Source: CAD feature listing. Evaluate the final solid. Frame: model axes, mm. Give positions to 0.01 mm unless a question says otherwise; leave off trailing zeros. Order: outer loops, then holes, each group sorted by start corner. A loop starts at its lowest first (then second) coordinate and runs counter-clockwise, first axis right, second up. Notation, with made-up numbers: (51.5, 56) - (62.5, 56) arc R25 cw to (62.5, 94) - close; hole circle Ø10 at (41, 42.5). An arc over 180 degrees is marked (long way). Write each question's results on one line, items separated by ' | '. Start each with the question number.
Item 1: Section C-C on y = 1139. Output: boundary loops of the cut face in (x, z), and give its area (3 significant figures).
Item 2: Contact query for flat-ended pins moving along their axis: pin 1 Ø2 at (x, y) = (5.5, 1030.5) entering from +Z; pin 2 Ø1.2 at (x, y) = (0.5, 1124) entering from -Z; pin 3 Ø1.2 at (y, z) = (1205.5, -1) entering from -X; pin 4 Ø1.6 at (x, z) = (1, -10) entering from +Y. Output: stop coordinate, or through.
Item 3: Section B-B on z = -8.75. Output: boundary loops of the cut face in (x, y), and give its area (4 significant figures).
Item 4: Section A-A on x = 4.5. Output: boundary loops of the cut face in (y, z).
Item 5: Line query: line 1 along X through (y, z) = (980, -14.5); line 2 along Z through (x, y) = (12, 1135.5); line 3 along Y through (x, z) = (4.5, -1). Output: solid intervals per line, ascending.
```python
from build123d import *

# Parameters (mm, degrees)
SKETCH1_W                   = 17
SKETCH1_H                   = 17
BOSS_EXTRUDE1_DEPTH         = 1220
CUT_EXTRUDE1_START          = -20
SKETCH2_W                   = 20
SKETCH2_H                   = 20
CUT_EXTRUDE1_DEPTH          = 10
CUT_EXTRUDE2_DEPTH          = 15
SKETCH4_W                   = 3
SKETCH4_H                   = 10
CUT_EXTRUDE3_DEPTH          = 10
SKETCH_PATTERN1_START       = -20
SKETCH_PATTERN1_DEPTH       = 15
SKETCH_PATTERN1_2_OUTLINE_W = 1.5
SKETCH_PATTERN1_2_OUTLINE_H = 10
SKETCH_PATTERN1_2_DEPTH     = 3
SKETCH6_W                   = 20
SKETCH6_H                   = 785
CUT_EXTRUDE4_DEPTH          = 1221.327824808


# Read off the part's stored shape, not the designer's step: Sketch-Pattern1
with BuildPart() as part:
    # Sketch1 → Boss-Extrude1 (new body)
    with BuildSketch(Plane(origin=(0, 0, 0), x_dir=(1, 0, 0), z_dir=(0, 1, 0))):
        with BuildLine():
            Line((0.5, 0), (19.5, 0))
            ThreePointArc((19.5, 0), (19.853553391, 0.146446609), (20, 0.5))
            Line((20, 0.5), (20, 19.5))
            ThreePointArc((20, 19.5), (19.853553391, 19.853553391), (19.5, 20))
            Line((19.5, 20), (0.5, 20))
            ThreePointArc((0.5, 20), (0.146446609, 19.853553391), (0, 19.5))
            Line((0, 19.5), (0, 0.5))
            ThreePointArc((0, 0.5), (0.146446609, 0.146446609), (0.5, 0))
        make_face()
        with Locations((10, 10)):
            Rectangle(SKETCH1_W, SKETCH1_H, mode=Mode.SUBTRACT)
    extrude(amount=BOSS_EXTRUDE1_DEPTH)

    # Sketch2 → Cut-Extrude1 (cut)
    with BuildSketch(Plane(origin=(20, 0, 0), x_dir=(0, 0, -1), z_dir=(1, 0, 0)).offset(CUT_EXTRUDE1_START)):
        with Locations((10, 1210)):
            Rectangle(SKETCH2_W, SKETCH2_H)
        with Locations((10, 10)):
            Rectangle(SKETCH2_W, SKETCH2_H)
    extrude(amount=CUT_EXTRUDE1_DEPTH, mode=Mode.SUBTRACT)

    # Sketch3 → Cut-Extrude2 (cut)
    with BuildSketch(Plane(origin=(0, 0, -20), x_dir=(-1, 0, 0), z_dir=(0, 0, -1))):
        Polygon((-15, 1115), (0, 1115), (0, 1120), (-9, 1120), (-9, 1130), (0, 1130), (0, 1135), (-15, 1135), align=None)
    extrude(amount=-CUT_EXTRUDE2_DEPTH, mode=Mode.SUBTRACT)

    # Sketch4 → Cut-Extrude3 (cut)
    with BuildSketch(Plane.ZY):
        with Locations((-18.5, 1125)):
            Rectangle(SKETCH4_W, SKETCH4_H)
    extrude(amount=-CUT_EXTRUDE3_DEPTH, mode=Mode.SUBTRACT)

    # Sketch-Pattern1 outline → Sketch-Pattern1 (cut)
    with BuildSketch(Plane.XY.offset(SKETCH_PATTERN1_START)):
        Polygon((15, 85), (15, 105), (0, 105), (0, 100), (1.5, 100), (1.5, 90), (0, 90), (0, 85), align=None)
        Polygon((1.5, 330), (1.5, 320), (0, 320), (0, 315), (15, 315), (15, 335), (0, 335), (0, 330), align=None)
        Polygon((1.5, 500), (1.5, 490), (0, 490), (0, 485), (15, 485), (15, 505), (0, 505), (0, 500), align=None)
        Polygon((1.5, 730), (1.5, 720), (0, 720), (0, 715), (15, 715), (15, 735), (0, 735), (0, 730), align=None)
        Polygon((1.5, 900), (1.5, 890), (0, 890), (0, 885), (15, 885), (15, 905), (0, 905), (0, 900), align=None)
    extrude(amount=SKETCH_PATTERN1_DEPTH, mode=Mode.SUBTRACT)

    # Sketch-Pattern1 2 outline → Sketch-Pattern1 2 (cut)
    with BuildSketch(Plane.XY.offset(SKETCH_PATTERN1_START)):
        with Locations((0.75, 95)):
            Rectangle(SKETCH_PATTERN1_2_OUTLINE_W, SKETCH_PATTERN1_2_OUTLINE_H)
        with Locations((0.75, 325)):
            Rectangle(SKETCH_PATTERN1_2_OUTLINE_W, SKETCH_PATTERN1_2_OUTLINE_H)
        with Locations((0.75, 495)):
            Rectangle(SKETCH_PATTERN1_2_OUTLINE_W, SKETCH_PATTERN1_2_OUTLINE_H)
        with Locations((0.75, 725)):
            Rectangle(SKETCH_PATTERN1_2_OUTLINE_W, SKETCH_PATTERN1_2_OUTLINE_H)
        with Locations((0.75, 895)):
            Rectangle(SKETCH_PATTERN1_2_OUTLINE_W, SKETCH_PATTERN1_2_OUTLINE_H)
    extrude(amount=SKETCH_PATTERN1_2_DEPTH, mode=Mode.SUBTRACT)

    # Sketch6 → Cut-Extrude4 (cut, through all)
    with BuildSketch(Plane(origin=(0, 0, -20), x_dir=(-1, 0, 0), z_dir=(0, 0, -1))):
        with Locations((-10, 392.5)):
            Rectangle(SKETCH6_W, SKETCH6_H)
    extrude(amount=-CUT_EXTRUDE4_DEPTH, mode=Mode.SUBTRACT)


solid = part.part
```
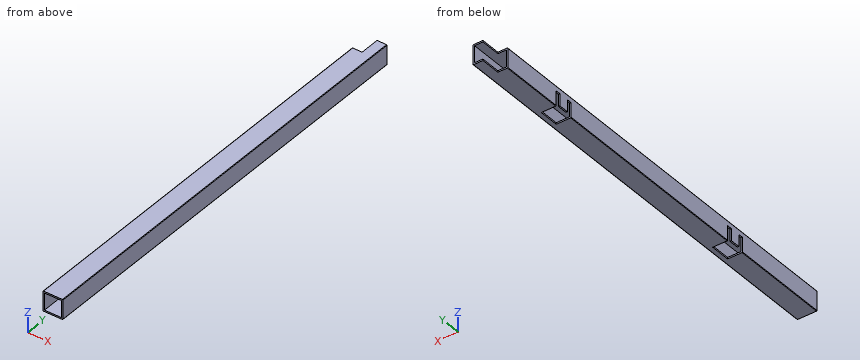
Evaluation:
1) outline: (0, -19.5) arc R0.5 ccw to (0.5, -20) - (19.5, -20) arc R0.5 ccw to (20, -19.5) - (20, -0.5) arc R0.5 ccw to (19.5, 0) - (0.5, 0) arc R0.5 ccw to (0, -0.5) - close; hole (1.5, -18.5) - (18.5, -18.5) - (18.5, -1.5) - (1.5, -1.5) - close | area: 111 mm^2
2) pin 1: stops at z = 0 | pin 2: stops at z = -17 | pin 3: stops at x = 10 | pin 4: stops at y = 1200
3) outline: (0, 785) - (1.5, 785) - (1.5, 885) - (0, 885) - close; (0, 890) - (1.5, 890) - (1.5, 900) - (0, 900) - close; (0, 905) - (1.5, 905) - (1.5, 1115) - (0, 1115) - close; (0, 1120) - (1.5, 1120) - (1.5, 1130) - (0, 1130) - close; (0, 1135) - (1.5, 1135) - (1.5, 1200) - (0, 1200) - close; (18.5, 785) - (20, 785) - (20, 1220) - (18.5, 1220) - close | area: 1,245 mm^2
4) outline: (785, -20) - (885, -20) - (885, -18.5) - (785, -18.5) - close; (785, -1.5) - (1200, -1.5) - (1200, 0) - (785, 0) - close; (905, -20) - (1115, -20) - (1115, -18.5) - (905, -18.5) - close; (1135, -20) - (1200, -20) - (1200, -18.5) - (1135, -18.5) - close
5) line 1: x = 0 to 1.5, 18.5 to 20 | line 2: z = -20 to -18.5, -1.5 to 0 | line 3: y = 785 to 1200
